Source: CAD feature listing. Evaluate the final solid. Frame: model axes, mm. Face numbers are marked on the shaded views. Round coordinates to 2 decimals unless told otherwise and drop trailing zeros. Write each loop counter-clockwise with the first axis right and the second up, starting at its lowest first coordinate (ties: lowest second). Pieces come first, ordered by that corner, then holes. Notation, with made-up numbers: M -15,81.5 L 31,81.5 A28 cw 31,109.5 Z; hole C 34.25,-17 d6. An arc over 180 degrees is marked long. Answer in a Markdown table with one row per item. Add a question column.
Item 1: Cut plane B-B on y = 0.95. Give the number of separate pieces and of enclosed holes in the cut face, and give its area (3 significant figures).
Item 2: Contact query for a flat-ended pin moving along its axis: pin 1 (1 mm diameter, centred on x = 4, y = 2, fed in from +Z). Output: stop coordinate, or through.
Item 3: Mould query, pull axis Y, two halves, no side actions, for the marked faces 1 and 2. Classes: released by +Y, released by -Y, zero draft, split by the parting line, or undercut.
Item 4: Cut plane C-C on x = -25.4. Return loops of the section in (y, z) (1 decimal).
Item 5: Cut plane A-A on z = 13.97. Return loops of the section in (x, y) (1 decimal), and give its area (3 significant figures).
Item 6: Material intervals for probe 1 along X at (y, z) = (1.7, -6.35); probe 2 along X at (y, z) = (1, 13.97); probe 3 along X at (y, z) = (0.2, 23.5), sorted ascending.
Item 7: Cut plane D-D on z = -6.35. Return loops of the section in (x, y) (1 decimal).
from build123d import *

# Parameters (mm, degrees)
SKETCH1_R           = 1.5875
BOSS_EXTRUDE1_DEPTH = 3.175
FILLET1_R           = 1.778


with BuildPart() as part:
    # Sketch1 → Boss-Extrude1 (new body)
    with BuildSketch(Plane(origin=(0, 0, 0), x_dir=(1, 0, 0), z_dir=(0, 1, 0))):
        Polygon((38.1, 12.7), (-38.1, 12.7), (-38.1, -42.545), (-12.7, -42.545), (-12.7, 0), (12.7, 0), (12.7, -42.545), (38.1, -42.545), align=None)
        with Locations(Location((-25.4, -13.97, 0), (0, 0, 270))):
            Circle(SKETCH1_R, mode=Mode.SUBTRACT)
        with Locations(Location((25.4, -13.97, 0), (0, 0, 90))):
            Circle(SKETCH1_R, mode=Mode.SUBTRACT)
        with Locations(Location((-12.7, 6.35, 0), (0, 0, 270))):
            Circle(SKETCH1_R, mode=Mode.SUBTRACT)
        with Locations(Location((12.7, 6.35, 0), (0, 0, 90))):
            Circle(SKETCH1_R, mode=Mode.SUBTRACT)
    extrude(amount=BOSS_EXTRUDE1_DEPTH)

    # Fillet1
    fillet1_edges = [part.edges().sort_by_distance(p)[0] for p in [
        (12.7, 1.5875, 0),
        (-12.7, 1.5875, 0),
    ]]
    fillet(fillet1_edges, radius=FILLET1_R)


solid = part.part
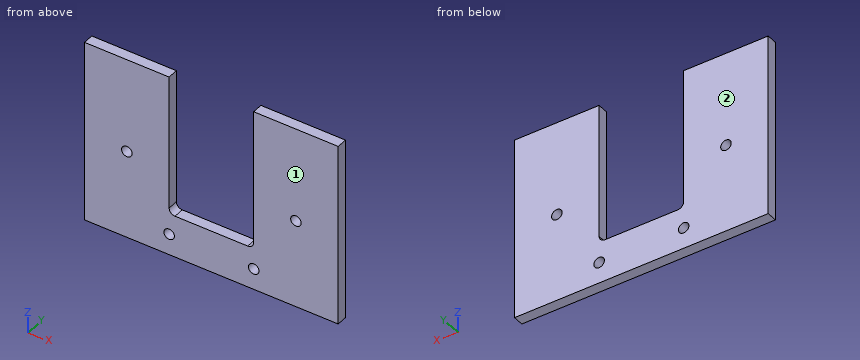
Results below:
| question | item | result |
|---|---|---|
| 1 | separate pieces | 1 |
| 1 | enclosed holes | 4 |
| 1 | area | 3,100 mm2 |
| 2 | pin 1 | z = 0 |
| 3 | face 1 | released by -Y |
| 3 | face 2 | released by +Y |
| 4 | outline | M 0,-12.7 L 3.2,-12.7 L 3.2,12.4 L 0,12.4 Z; M 0,15.6 L 3.2,15.6 L 3.2,42.5 L 0,42.5 Z |
| 5 | outline | M -38.1,0 L -27,0 L -27,3.2 L -38.1,3.2 Z; M -23.8,0 L -12.7,0 L -12.7,3.2 L -23.8,3.2 Z; M 12.7,0 L 23.8,0 L 23.8,3.2 L 12.7,3.2 Z; M 27,0 L 38.1,0 L 38.1,3.2 L 27,3.2 Z |
| 5 | area | 141 mm2 |
| 6 | probe 1 | -38.1 to -14.29, -11.11 to 11.11, 14.29 to 38.1 |
| 6 | probe 2 | -38.1 to -26.99, -23.81 to -12.7, 12.7 to 23.81, 26.99 to 38.1 |
| 6 | probe 3 | -38.1 to -12.7, 12.7 to 38.1 |
| 7 | outline | M -38.1,0 L -14.3,0 L -14.3,3.2 L -38.1,3.2 Z; M -11.1,0 L 11.1,0 L 11.1,3.2 L -11.1,3.2 Z; M 14.3,0 L 38.1,0 L 38.1,3.2 L 14.3,3.2 Z |
